Geometry check sheet. Reference: the model listing, model coordinates, mm. Face numbers are marked on the shaded views. A direction names the side the tool comes from. Give positions to 0.01 mm unless a question says otherwise; leave off trailing zeros. Loops run counter-clockwise (first coordinate to the right, second up) from the corner with the lowest first, then second, coordinate; pieces in that order, holes last. Notation, with made-up numbers: (-38, 5.25) -> (19, 5.25) arc R15 ccw to (19, 32.25) -> close; hole circle Ø5 at (16, 73). An arc over 180 degrees is marked (long way). Answer as a JSON object with one key per item and string values.
from build123d import *

# Parameters (mm, degrees)
F0_R     = 7.9375
F2_DEPTH = 25.4
F1_R     = 12.7
F3_DEPTH = 6.35
F4_R     = 5.08
F5_R     = 2.032
F6_R     = 1.27
F7_DEPTH = 38.1


with BuildPart() as f2:
    # F0 (on Top) → F2 (new body)
    with BuildSketch(Plane.XY):
        Circle(F0_R)
    extrude(amount=F2_DEPTH)

    # F1 (on Top) → F3 (join)
    with BuildSketch(Plane.XY):
        Circle(F1_R)
    extrude(amount=F3_DEPTH)

    # F4
    f4_edges = [f2.edges().sort_by_distance(p)[0] for p in [
        (-7.9375, 0, 25.4),
    ]]
    fillet(f4_edges, radius=F4_R)

    # F5
    f5_edges = [f2.edges().sort_by_distance(p)[0] for p in [
        (-12.7, 0, 6.35),
    ]]
    fillet(f5_edges, radius=F5_R)

    # F6 (on face) → F7 (cut)
    with BuildSketch(Plane.XY.offset(25.4)):
        Circle(F6_R)
    extrude(amount=-F7_DEPTH, mode=Mode.SUBTRACT)


solid = f2.part
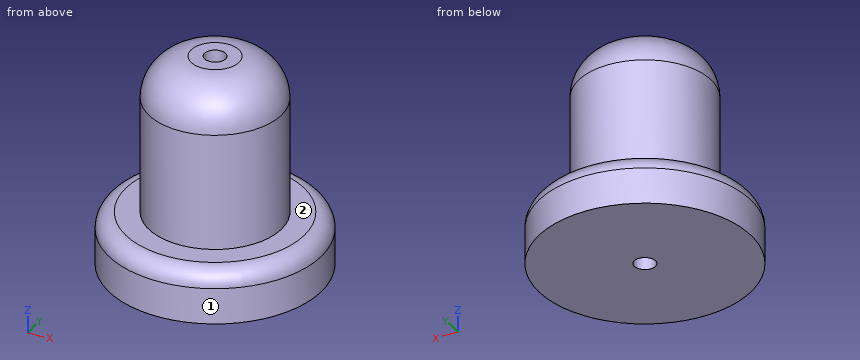
1) Material ranges on line 1 along Y through (x, z) = (0, 7.25); line 2 along Z through (x, y) = (-4.5, -7.75); line 3 along X through (y, z) = (-1, 5), recorded low to high. Write a range as from..to.
Geometry check:
{"line 1": "y = -7.94..-1.27, 1.27..7.94", "line 2": "z = 0..6.35", "line 3": "x = -12.54..-0.78, 0.78..12.54"}
2) Section check A-A on z = 3. Record the cut outline in (x, y).
Geometry check:
{"outline": "circle Ø25.4 at (0, 0); hole circle Ø2.54 at (0, 0)"}
3) Tool access check on the marked faces 1 and 2. Record the directions out of +Z, -Z, +X, -X, +Y, -Y that give a thin tool (end or side, any length) a straight path to the whole face; none if there is none.
Geometry check:
{"face 1": "+Z, -Z", "face 2": "+Z"}
4) Depth check by flat-ended pin: P1, Ø2, axis at x = 4.5, z = 21.5, coming from the -Y side; P2, Ø2, axis at y = -8.5, z = 3.5, coming from the -X side; P3, Ø1, axis at y = 3, z = 16, coming from the +X side. Enter the tip coordinate at first touch or a pass-through.
Geometry check:
{"P1": "stops at y = -7.02", "P2": "stops at x = -10.25", "P3": "stops at x = 7.53"}
